Answer from the drawing. Dimensions are ordinates in mm from the lowest x, y and z of the part. Round coordinates to 2 decimals unless told otherwise and drop trailing zeros. Write each loop counter-clockwise with the first axis right and the second up, starting at its lowest first coordinate (ties: lowest second). Pieces come first, ordered by that corner, then holes. Notation, with made-up numbers: (72, -23) -> (108, -23) arc R21 cw to (108, 12) -> close; hole circle Ø3 at (80.25, 44.5). An arc over 180 degrees is marked (long way). Return JSON: item names as keys, results as strings. Group by question number.
(1) A cutting plane is placed at D-D on x = 2.5. Give the vertices of the cut face in (y, z).
(2) A cutting plane is placed at C-C on z = 1.35. Give the vertices of the cut face in (x, y).
(3) Given pin 1 (1.5 mm diameter, centred on y = 10.5, z = 0.5, fed in from +X); pin 2 (1 mm diameter, centred on x = 3, z = 1.5, fed in from -Y), each flat-ended and moving along its own axis, determine where each tip first touches the part or whether it passes through.
(4) A cutting plane is placed at A-A on y = 6. Give the vertices of the cut face in (x, z), then the cut area to 3 significant figures.
(5) Straight lines are drawn through the part: line 1 (Y direction, x = 6, z = 0.2); line 2 (Y direction, x = 6, z = 2.7); line 3 (Z direction, x = 1, y = 6.5). For each, find the intervals that lie inside material, in ascending order.
(6) The mould has two halves that part along X. Classify the marked faces 1, 2, 3 and 4: released by +X, released by -X, zero draft, split by the parting line, or undercut.
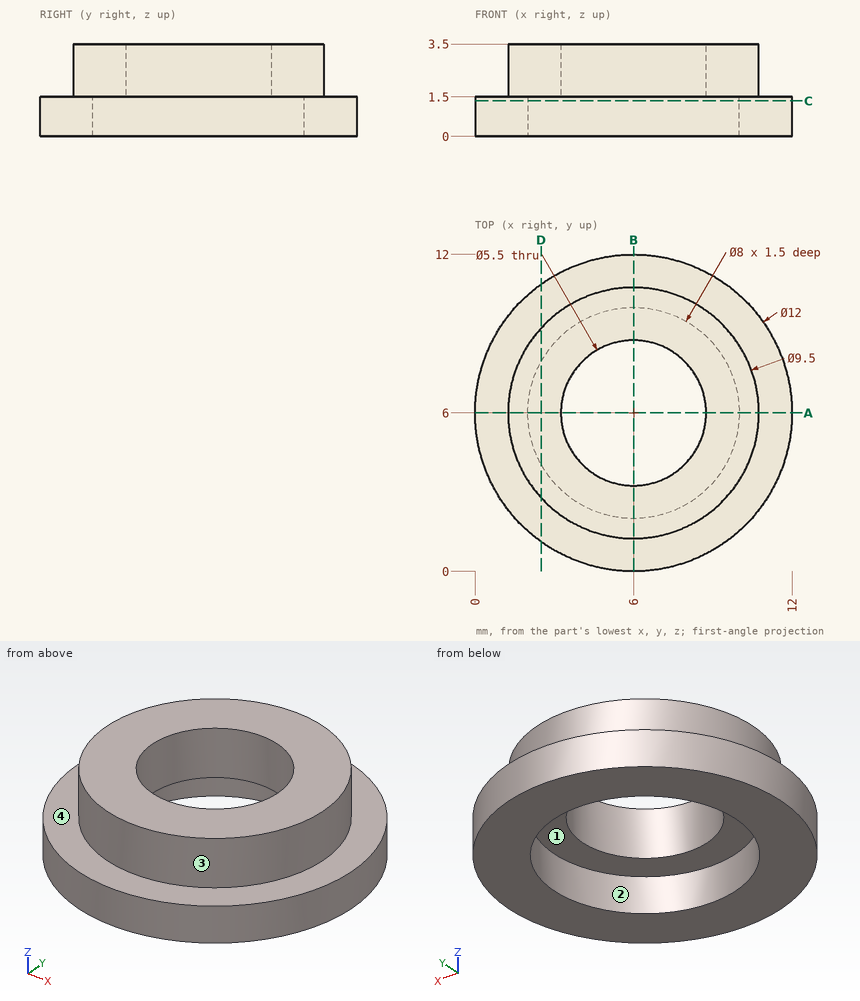
Checks:
{
 "1": {"outline": "(1.13, 0) -> (4.06, 0) -> (4.06, 1.5) -> (7.94, 1.5) -> (7.94, 0) -> (10.87, 0) -> (10.87, 1.5) -> (9.21, 1.5) -> (9.21, 3.5) -> (2.79, 3.5) -> (2.79, 1.5) -> (1.13, 1.5) -> close"},
 "2": {"outline": "circle Ø12 at (6, 6); hole circle Ø8 at (6, 6)"},
 "3": {"pin 1": "stops at x = 10.68", "pin 2": "stops at y = 0.55"},
 "4": {"outline": "(0, 0) -> (2, 0) -> (2, 1.5) -> (3.25, 1.5) -> (3.25, 3.5) -> (1.25, 3.5) -> (1.25, 1.5) -> (0, 1.5) -> close; (8.75, 1.5) -> (10, 1.5) -> (10, 0) -> (12, 0) -> (12, 1.5) -> (10.75, 1.5) -> (10.75, 3.5) -> (8.75, 3.5) -> close", "area": "14.0 mm^2"},
 "5": {"line 1": "y = 0 to 2, 10 to 12", "line 2": "y = 1.25 to 3.25, 8.75 to 10.75", "line 3": "z = 0 to 1.5"},
 "6": {"face 1": "undercut", "face 2": "undercut", "face 3": "split by the parting line", "face 4": "zero draft"}
}
